```python
from build123d import *

# Parameters (mm, degrees)
SKETCH_1_W                  = 28
SKETCH_1_H                  = 15
EXTRUDE_1_DEPTH             = 5
EXTRUDE_2_DEPTH             = 13
EXTRUDE_2_DIRECTION_2_REACH = 34.156
CUT_EXTRUDE_1_DEPTH         = 53.098032867
SKETCH_8_W                  = 41
SKETCH_8_H                  = 40
EXTRUDE_3_DEPTH             = 2.5
SKETCH_4_R                  = 1.4
CUT_EXTRUDE_2_DEPTH         = 7
SKETCH_5_R                  = 1.65
CUT_EXTRUDE_3_DEPTH         = 45.800573211
SKETCH_6_W                  = 33.531677497
SKETCH_6_H                  = 7.773496997
CUT_EXTRUDE_4_DEPTH         = 11
FILLET_1_R                  = 2
CUT_EXTRUDE_5_DEPTH         = 44.302936624
SKETCH_10_W                 = 2
SKETCH_10_H                 = 11.556486704
CUT_EXTRUDE_6_DEPTH         = 6
CUT_EXTRUDE_8_DEPTH         = 8
CUT_EXTRUDE_9_DEPTH         = 12
FILLET_2_R                  = 3
EXTRUDE_4_DEPTH             = 5


with BuildPart() as part:
    # 草图1 → 凸台-拉伸1 (new body)
    with BuildSketch(Plane(origin=(0, 0, 0), x_dir=(1, 0, 0), z_dir=(0, 1, 0))):
        with Locations((14, 7.5)):
            Rectangle(SKETCH_1_W, SKETCH_1_H)
    extrude(amount=EXTRUDE_1_DEPTH)

    # 草图2 → 凸台-拉伸2 (add)
    with BuildSketch(Plane.ZY):
        Polygon((4.811400568, -9.800725827), (-29.294206006, 11.099216762), (-27.987959594, 13.230817173), (-14.556486704, 5), (0, 5), (0, 0), (0, -3.920226525), (6.11764698, -7.669125416), align=None)
    extrude(amount=EXTRUDE_2_DEPTH)

    # 凸台-拉伸2 direction 2: up to this face of the body (flat: up to its plane)
    extrude_2_direction_2_end = Plane(part.part.faces().sort_by_distance((28, 2.5, -7.5))[0])
    # 草图2 → 凸台-拉伸2 direction 2 (add, up to the picked face)
    with BuildSketch(Plane.ZY, mode=Mode.PRIVATE) as extrude_2_direction_2_sk1:
        Polygon((4.811400568, -9.800725827), (-29.294206006, 11.099216762), (-27.987959594, 13.230817173), (-14.556486704, 5), (0, 5), (0, 0), (0, -3.920226525), (6.11764698, -7.669125416), align=None)
    extrude_2_direction_2_tool1 = split(extrude(extrude_2_direction_2_sk1.sketch, amount=-EXTRUDE_2_DIRECTION_2_REACH, mode=Mode.PRIVATE), bisect_by=extrude_2_direction_2_end, keep=Keep.BOTH, mode=Mode.PRIVATE)
    add(extrude_2_direction_2_tool1.solids().sort_by(Axis((0, 1.837688, -8.936549), (1, 0, 0)))[0])

    # 草图3 → 切除-拉伸1 (cut, through all)
    with BuildSketch(Plane.ZY.offset(13)):
        Polygon((-15, 0), (-11.181930407, 0), (-15, 2.339716056), align=None)
    extrude(amount=-CUT_EXTRUDE_1_DEPTH, mode=Mode.SUBTRACT)

    # 草图8 → 凸台-拉伸3 (add)
    with BuildSketch(Plane(origin=(0, -4.981586473, -3.052720117), x_dir=(1, 0, 0), z_dir=(0, -0.8526401643540905, -0.5224985647159519))):
        with Locations((7.5, -10.776741451)):
            Rectangle(SKETCH_8_W, SKETCH_8_H)
    extrude(amount=EXTRUDE_3_DEPTH)

    # 草图4 → 切除-拉伸2 (cut)
    with BuildSketch(Plane(origin=(0, -7.113186884, -4.358966529), x_dir=(1, 0, 0), z_dir=(0, -0.8526401643540905, -0.5224985647159519))):
        with Locations(Location((-9.945229951, 6.723258549, 0), (0, 0, 270))):
            Circle(SKETCH_4_R)
        with Locations(Location((25.054770049, 6.723258549, 0), (0, 0, 270))):
            Circle(SKETCH_4_R)
        with Locations(Location((25.054770049, -28.276741451, 0), (0, 0, 270))):
            Circle(SKETCH_4_R)
        with Locations(Location((-9.945229951, -28.276741451, 0), (0, 0, 270))):
            Circle(SKETCH_4_R)
    extrude(amount=-CUT_EXTRUDE_2_DEPTH, mode=Mode.SUBTRACT)

    # 草图5 → 切除-拉伸3 (cut, through all)
    with BuildSketch(Plane(origin=(0, 5, 0), x_dir=(1, 0, 0), z_dir=(0, 1, 0))):
        with Locations(Location((10.5, 9.8, 0), (0, 0, 270))):
            Circle(SKETCH_5_R)
        with Locations(Location((0.5, 9.8, 0), (0, 0, 270))):
            Circle(SKETCH_5_R)
    extrude(amount=-CUT_EXTRUDE_3_DEPTH, mode=Mode.SUBTRACT)

    # 草图6 → 切除-拉伸4 (cut)
    with BuildSketch(Plane(origin=(0, 2, 0), x_dir=(1, 0, 0), z_dir=(0, 1, 0))):
        with Locations((7.374838624, 9.340740808)):
            Rectangle(SKETCH_6_W, SKETCH_6_H)
    extrude(amount=-CUT_EXTRUDE_4_DEPTH, mode=Mode.SUBTRACT)

    # 圆角1
    fillet_1_edges = [part.edges().sort_by_distance(p)[0] for p in [
        (28, 11.099216762, -29.294206006),
        (28, -9.800725827, 4.811400568),
        (-13, -9.800725827, 4.811400568),
        (-13, 11.099216762, -29.294206006),
    ]]
    fillet(fillet_1_edges, radius=FILLET_1_R)

    # 草图9 → 切除-拉伸5 (cut, through all)
    with BuildSketch(Plane(origin=(0, -2.849986062, -1.746473705), x_dir=(1, 0, 0), z_dir=(0, 0.8526401643540904, 0.5224985647159519))):
        with BuildLine():
            Line((-8.286917555, -9.223258549), (23.396457654, -9.223258549))
            ThreePointArc((23.396457654, -9.223258549), (22.073973693, -6.384358742), (24, -3.914796311))
            Line((24, -3.914796311), (24, -2.048312733))
            Line((24, -2.048312733), (-9, -2.048312733))
            Line((-9, -2.048312733), (-9, -3.876059866))
            ThreePointArc((-9, -3.876059866), (-6.971555183, -6.326700388), (-8.286917555, -9.223258549))
        make_face()
        with BuildLine():
            Line((-9, 19.02393804), (-9, 15.02393804))
            Line((-9, 15.02393804), (24, 15.02393804))
            Line((24, 15.02393804), (24, 19.02393804))
            Line((24, 19.02393804), (24, 25.468279213))
            ThreePointArc((24, 25.468279213), (22.073973693, 27.937841645), (23.396457654, 30.776741451))
            Line((23.396457654, 30.776741451), (-8.286917555, 30.776741451))
            ThreePointArc((-8.286917555, 30.776741451), (-6.971555183, 27.880183291), (-9, 25.429542768))
            Line((-9, 25.429542768), (-9, 19.02393804))
        make_face()
    extrude(amount=-CUT_EXTRUDE_5_DEPTH, mode=Mode.SUBTRACT)

    # 草图10 → 切除-拉伸6 (cut)
    with BuildSketch(Plane(origin=(0, 5, 0), x_dir=(1, 0, 0), z_dir=(0, 1, 0))):
        with Locations((5.501092332, 4.778243352)):
            Rectangle(SKETCH_10_W, SKETCH_10_H)
    extrude(amount=-CUT_EXTRUDE_6_DEPTH, mode=Mode.SUBTRACT)

    # 草图11 → 切除-拉伸8 (cut)
    with BuildSketch(Plane.ZY.offset(13)):
        Polygon((0, -3.920226525), (-14.556486704, 5), (0, 5), align=None)
    extrude(amount=-CUT_EXTRUDE_8_DEPTH, mode=Mode.SUBTRACT)

    # 草图12 → 切除-拉伸9 (cut)
    with BuildSketch(Plane(origin=(28, 0, 0), x_dir=(0, 0, -1), z_dir=(1, 0, 0))):
        Polygon((14.556486704, 5), (0, -3.920226525), (0, 5), align=None)
    extrude(amount=-CUT_EXTRUDE_9_DEPTH, mode=Mode.SUBTRACT)

    # 圆角2
    fillet_2_edges = [part.edges().sort_by_distance(p)[0] for p in [
        (11.250546166, 5, 0),
        (-0.249453834, 5, 0),
    ]]
    fillet(fillet_2_edges, radius=FILLET_2_R)

    # 草图13 → 凸台-拉伸4 (add)
    with BuildSketch(Plane(origin=(0, -7.113186884, -4.358966529), x_dir=(1, 0, 0), z_dir=(0, -0.8526401643540905, -0.5224985647159519))):
        with BuildLine():
            Line((27.203064282, -17.882084245), (29.512557602, -17.882084245))
            ThreePointArc((29.512557602, -17.882084245), (32.512557602, -20.882084245), (29.512557602, -23.882084245))
            Line((29.512557602, -23.882084245), (27.203064282, -23.882084245))
            Line((27.203064282, -23.882084245), (27.203064282, -25.882084245))
            Line((27.203064282, -25.882084245), (29.512557602, -25.882084245))
            ThreePointArc((29.512557602, -25.882084245), (34.512557602, -20.882084245), (29.512557602, -15.882084245))
            Line((29.512557602, -15.882084245), (27.203064282, -15.882084245))
            Line((27.203064282, -15.882084245), (27.203064282, -17.882084245))
        make_face()
    extrude(amount=-EXTRUDE_4_DEPTH)


solid = part.part
```
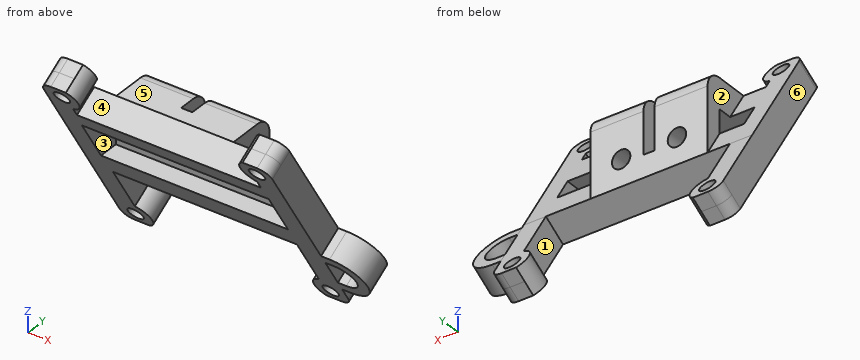
Check sheet for the modelled part. Datum: model origin and axes. Units: mm. Face numbers are marked on the shaded views. A direction names the side the tool comes from. Round coordinates to 2 decimals unless told otherwise and drop trailing zeros. Order: outer loops, then holes, each group sorted by start corner. A loop starts at its lowest first (then second) coordinate and runs counter-clockwise, first axis right, second up. Notation, with made-up numbers: (84.5, 2) -> (141.5, 2) arc R32 ccw to (141.5, 29) -> close; hole circle Ø8 at (80.5, -18.75). An arc over 180 degrees is marked (long way). One line per item, written item: value. Start each with the question number.
Q1. Mould release check, pull along X, two halves, no side actions. Record for the marked faces 4, 5 and 6: pulls with the +X half, pulls with the -X half, needs draft (parallel to the pull), parting line crosses it, or undercut.
Q2. Set-up check for the marked faces 1, 2 and 3: record each of +Z, -Z, +X, -X, +Y, -Y from which the full face is reachable in a straight line by a thin tool's end or side.
Q3. Cross-section at A-A (x = 0.5). Record the boundary of the cut face in (y, z).
Q4. Cross-section at C-C (z = -12.5). Record the boundary of the cut face in (x, y).
Q5. Cross-section at D-D (x = 19.5). Record the boundary of the cut face in (y, z), and give its area (3 significant figures).
Q6. Thickness scan on line 1 (X direction, y = 3.25, z = -9.8); line 2 (X direction, y = 11, z = -26); line 3 (Y direction, x = -2, z = -10.5). Record the ranges inside material, lowest first.
Q7. Cross-section at B-B (z = -7). Record the boundary of the cut face in (x, y), and give its area (3 significant figures).
Q8. Gauge pin test, flat ends, axial feed: pin 1 Ø2 at (x, y) = (7.5, 5.5) entering from +Z; pin 2 Ø4.5 at (x, z) = (0.5, -9.8) entering from -Y; pin 3 Ø2.5 at (x, y) = (12, -4) entering from -Z. Record the tip position at first contact, or that the pin passes through.
Completed:
1. face 4: undercut
1. face 5: needs draft
1. face 6: pulls with the -X half
2. face 1: none
2. face 2: +Z, -X, +Y
2. face 3: -Y
3. outline: (-8.18, -2.61) -> (-6.44, -5.45) -> (2, -5.45) -> (2, -8.15) -> (5, -8.15) -> (5, -3) arc R3 ccw to (2, 0) -> (-3.92, 0) -> close; (-1.68, -13.23) -> (0.74, -17.17) -> (5, -14.56) -> (5, -11.45) -> (2, -11.45) -> (2, -13.23) -> close
4. outline: (-13, -2.12) -> (-9.39, -2.12) -> (-9.39, 2) -> (24.14, 2) -> (24.14, -2.12) -> (28, -2.12) -> (28, 3.74) -> (16, 3.74) -> (16, 5) -> (-5, 5) -> (-5, 3.74) -> (-13, 3.74) -> close
5. outline: (-8.18, -2.61) -> (-6.44, -5.45) -> (-0.58, -5.45) -> (-3.92, 0) -> close; (-1.68, -13.23) -> (0.74, -17.17) -> (5, -14.56) -> (2, -9.66) -> (2, -13.23) -> close
5. area: 43.7 mm²
6. line 1: x = -5 to -1.15, 2.15 to 4.5, 6.5 to 8.85, 12.15 to 16
6. line 2: x = -13 to -11.3, -8.59 to -6.97, 22.08 to 23.7, 26.41 to 28
6. line 3: y = 2 to 5
7. outline: (-13, -5.49) -> (-9.39, -5.49) -> (-9.39, 0.37) -> (-13, 0.37) -> close; (-5, 2) -> (4.5, 2) -> (4.5, 5) -> (-5, 5) -> close; (6.5, 2) -> (16, 2) -> (16, 5) -> (6.5, 5) -> close; (24.14, -5.49) -> (28, -5.49) -> (28, 0.37) -> (24.14, 0.37) -> close
7. area: 101 mm²
8. pin 1: stops at z = -1.34
8. pin 2: stops at y = 2
8. pin 3: stops at z = -5.45
